```python
from build123d import *

# Parameters (mm, degrees)
Y_KSEKLIK_EKSTR_ZYON1_DEPTH = 50
KES_EKSTR_ZYON1_REACH       = 94.844
IZIM2_R                     = 10
KES_EKSTR_ZYON2_DEPTH       = 77.329104323
KES_EKSTR_ZYON2_DEPTH_BACK  = 77.329104323
RADYUS1_R                   = 10
RADYUS2_R                   = 10


with BuildPart() as part:
    # Çizim1 → Yükseklik-Ekstrüzyon1 (new body)
    with BuildSketch(Plane.XY):
        Polygon((-57.23116586, -11.25748503), (-27.23116586, -11.25748503), (-27.23116586, 28.74251497), (-17.23116586, 28.74251497), (-17.23116586, 21.706586826), (-17.23116586, -21.25748503), (-67.23116586, -21.25748503), (-67.23116586, 21.706586826), (-67.23116586, 28.74251497), (-57.23116586, 28.74251497), align=None)
    extrude(amount=Y_KSEKLIK_EKSTR_ZYON1_DEPTH)

    # Çizim2 → Kes-Ekstrüzyon1 (cut, up to next)
    with BuildSketch(Plane(origin=(0, -11.25748503, 0), x_dir=(1, 0, 0), z_dir=(0, 1, 0)), mode=Mode.PRIVATE) as kes_ekstr_zyon1_sk1:
        with Locations(Location((-42.23116586, -25, 0), (0, 0, 270))):
            Circle(IZIM2_R)
    kes_ekstr_zyon1_tool1 = extrude(kes_ekstr_zyon1_sk1.sketch, amount=-KES_EKSTR_ZYON1_REACH, mode=Mode.PRIVATE) & part.part
    add(kes_ekstr_zyon1_tool1.solids().sort_by_distance((-42.231166, -11.257485, 25))[0], mode=Mode.SUBTRACT)

    # Çizim3 → Kes-Ekstrüzyon2 (cut, two sides: drawn at the far end of the back side and taken through both)
    with BuildSketch(Plane(origin=(-17.23116586, 0, 0), x_dir=(0, 0, -1), z_dir=(1, 0, 0)).offset(-KES_EKSTR_ZYON2_DEPTH_BACK)):
        with BuildLine():
            Line((-35, 22.662565506), (-15, 22.662565506))
            ThreePointArc((-15, 22.662565506), (-10, 17.662565506), (-15, 12.662565506))
            Line((-15, 12.662565506), (-35, 12.662565506))
            ThreePointArc((-35, 12.662565506), (-40, 17.662565506), (-35, 22.662565506))
        make_face()
    extrude(amount=KES_EKSTR_ZYON2_DEPTH + KES_EKSTR_ZYON2_DEPTH_BACK, mode=Mode.SUBTRACT)

    # Radyus1
    radyus1_edges = [part.edges().sort_by_distance(p)[0] for p in [
        (-62.23116586, 28.74251497, 0),
        (-62.23116586, 28.74251497, 50),
    ]]
    fillet(radyus1_edges, radius=RADYUS1_R)

    # Radyus2
    radyus2_edges = [part.edges().sort_by_distance(p)[0] for p in [
        (-22.23116586, 28.74251497, 0),
        (-22.23116586, 28.74251497, 50),
    ]]
    fillet(radyus2_edges, radius=RADYUS2_R)


solid = part.part
```
Check sheet for the modelled part. Datum: model origin and axes. Units: mm. A direction names the side the tool comes from. Coordinates: 2 decimals unless noted, no trailing zeros. Order: outer loops, then holes, each group sorted by start corner. A loop starts at its lowest first (then second) coordinate and runs counter-clockwise, first axis right, second up. Notation, with made-up numbers: (-11.75, 72) -> (46.25, 72) arc R18 cw to (46.25, 106) -> close; hole circle Ø8 at (77.25, 5.25). An arc over 180 degrees is marked (long way). Write item = value, one per line. Start each with the question number.
1) Cross-section at A-A (y = 7). Enter the section's corners in (x, z), then the cut area to 3 significant figures.
2) Go/stop test with a flat-tipped pin: P1, Ø15, axis at x = -48.5, z = 28, coming from the +Y side. Record where the tip stops, or that it passes through.
3) Cross-section at B-B (z = 25). Enter the section's corners in (x, y), then the cut area to 3 significant figures.
4) Cross-section at C-C (x = -20.5). Enter the section's corners in (y, z).
5) Cross-section at D-D (y = -16.5). Enter the section's corners in (x, z), then the cut area to 3 significant figures.
6) Access from +Z, -Z, +X, -X, +Y, -Y to the whole of each face (thin tool, end or side, straight path). Record for faces 4 (the flat face through (-62, 22.663, 25)), 5 (the flat face through (-52.4, -11.257, 24.6)), 6 (the flat face through (-42, -14, 0)).
7) Material ranges on L1, parallel to X at y = -19, z = 25; L2, parallel to X at y = -0.5, z = 16; L3, parallel to Y at x = -60.5, z = 32, recorded low to high.
8) Mould release check, pull along Z, two halves, no side actions. Record for faces 1 (the cylindrical face through (-62.161, 25.735, 47.148)), 2 (the flat face through (-22, 22.663, 25)), 3 (the flat face through (-53, -21.257, 25)): +Z half, -Z half, draft (parallel to the pull), parting line (faces both ways), or undercut.
Ans:
q1.outline = (-67.23, 0) -> (-57.23, 0) -> (-57.23, 50) -> (-67.23, 50) -> close; (-27.23, 0) -> (-17.23, 0) -> (-17.23, 50) -> (-27.23, 50) -> close
q1.area = 1,000 mm²
q2.P1 = -11.26
q3.outline = (-67.23, -21.26) -> (-52.23, -21.26) -> (-52.23, -11.26) -> (-57.23, -11.26) -> (-57.23, 12.66) -> (-67.23, 12.66) -> close; (-67.23, 22.66) -> (-57.23, 22.66) -> (-57.23, 28.74) -> (-67.23, 28.74) -> close; (-32.23, -21.26) -> (-17.23, -21.26) -> (-17.23, 12.66) -> (-27.23, 12.66) -> (-27.23, -11.26) -> (-32.23, -11.26) -> close; (-27.23, 22.66) -> (-17.23, 22.66) -> (-17.23, 28.74) -> (-27.23, 28.74) -> close
q3.area = 900 mm²
q4.outline = (-21.26, 0) -> (18.74, 0) arc R10 ccw to (28.74, 10) -> (28.74, 40) arc R10 ccw to (18.74, 50) -> (-21.26, 50) -> close; hole (12.66, 15) arc R5 ccw to (22.66, 15) -> (22.66, 35) arc R5 ccw to (12.66, 35) -> close
q5.outline = (-67.23, 0) -> (-17.23, 0) -> (-17.23, 50) -> (-67.23, 50) -> close; hole circle Ø20 at (-42.23, 25)
q5.area = 2,190 mm²
q6.face_4 = +X, -X
q6.face_5 = +Z, -Z, +Y
q6.face_6 = -Z, +X, -X, +Y, -Y
q7.L1 = -67.23 to -52.23, -32.23 to -17.23
q7.L2 = -67.23 to -57.23, -27.23 to -17.23
q7.L3 = -21.26 to 12.66, 22.66 to 28.74
q8.face_1 = +Z half
q8.face_2 = undercut
q8.face_3 = draft
